Geometry: final body of the model. Coordinates: model frame, mm. Face numbers are marked on the shaded views. A direction names the side the tool comes from. Give positions to 0.01 mm unless a question says otherwise; leave off trailing zeros. Write each loop counter-clockwise with the first axis right and the second up, starting at its lowest first coordinate (ties: lowest second). Pieces come first, ordered by that corner, then holes. Notation, with made-up numbers: (1.25, -17) -> (36.25, -17) arc R15 ccw to (36.25, 11) -> close; hole circle Ø5 at (-2, 76). An arc over 180 degrees is marked (long way). Use CSV: the item, a comma, the result in double quotes. Start each with the question number.
1) Section C-C (x = -1.75). Output: boundary loops of the cut face in (y, z).
2) Section A-A (x = -12.5). Output: boundary loops of the cut face in (y, z).
3) Section D-D (z = -1). Output: boundary loops of the cut face in (x, y).
4) Set-up query: the marked faces 1 and 2. Return all of +Z, -Z, +X, -X, +Y, -Y with unobstructed straight access to the full face (end or side cutting, diameter ignored); none if empty.
5) Section B-B (y = 17.5). Output: boundary loops of the cut face in (x, z), plus the area to 3 significant figures.
6) Material intervals for line 1 (Y direction, x = -12.5, z = -2.3); line 2 (Y direction, x = -12.5, z = -1.5); line 3 (Z direction, x = -18.25, y = 10), sorted ascending. Write a range as [from, to].
7) Contact query for flat-ended pins moving along their axis: P1, Ø2, axis at x = -18, z = -9, coming from the +Y side; P2, Ø3, axis at x = -5.5, y = 11.5, coming from the -Z side; P3, Ø5, axis at x = -17.5, z = -2, coming from the +Y side; P4, Ø1, axis at x = -11, z = -6, coming from the +Y side. Output: stop coordinate, or through.
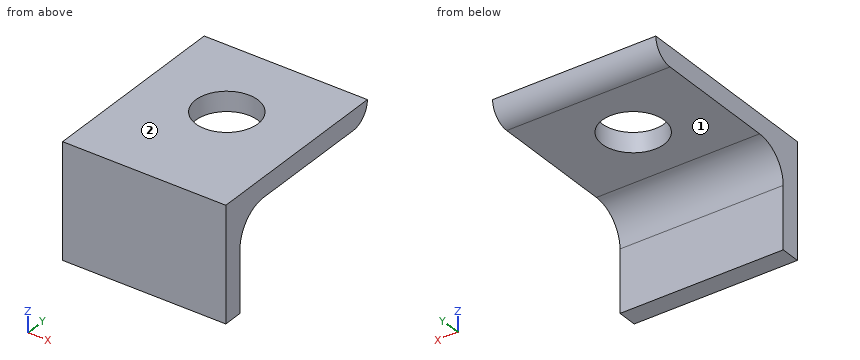
```python
from build123d import *

# Parameters (mm, degrees)
L_ANGLE_EQUAL_30X30X3_2_DEPTH  = 25
F_9_5_9_5_DIAMETER_HOLE1_D     = 9.5
F_9_5_9_5_DIAMETER_HOLE1_DEPTH = 18
F_9_5_9_5_DIAMETER_HOLE1_TIP   = 2.85408794
CUT_EXTRUDE1_REACH             = 51.244
SKETCH15_W                     = 25
SKETCH15_H                     = 12.5


with BuildPart() as part:
    # Sketch19 → L angle (equal) 30X30X3(2) (new body)
    with BuildSketch(Plane(origin=(-25, 0, 0), x_dir=(0, 0, -1), z_dir=(1, 0, 0))):
        with BuildLine():
            Line((0, 30), (0, 0))
            Line((0, 0), (30, 0))
            ThreePointArc((30, 0), (29.121320344, 2.121320344), (27, 3))
            Line((27, 3), (8, 3))
            ThreePointArc((8, 3), (4.464466094, 4.464466094), (3, 8))
            Line((3, 8), (3, 27))
            ThreePointArc((3, 27), (2.121320344, 29.121320344), (0, 30))
        make_face()
    extrude(amount=L_ANGLE_EQUAL_30X30X3_2_DEPTH)

    # Ø9.5 (9.5) Diameter Hole1
    with Locations(Plane(origin=(0, 0, -3), x_dir=(-1, 0, 0), z_dir=(0, 0, -1))):
        with Locations((12.5, 17.5)):
            Hole(F_9_5_9_5_DIAMETER_HOLE1_D / 2, depth=F_9_5_9_5_DIAMETER_HOLE1_DEPTH)
            with Locations((0, 0, -(F_9_5_9_5_DIAMETER_HOLE1_DEPTH + F_9_5_9_5_DIAMETER_HOLE1_TIP / 2))):  # 118° drill point
                Cone(0, F_9_5_9_5_DIAMETER_HOLE1_D / 2, F_9_5_9_5_DIAMETER_HOLE1_TIP, mode=Mode.SUBTRACT)

    # Sketch15 → Cut-Extrude1 (cut, up to next)
    with BuildSketch(Plane.XZ, mode=Mode.PRIVATE) as cut_extrude1_sk1:
        with Locations((-12.5, -23.75)):
            Rectangle(SKETCH15_W, SKETCH15_H)
    cut_extrude1_tool1 = extrude(cut_extrude1_sk1.sketch, amount=-CUT_EXTRUDE1_REACH, mode=Mode.PRIVATE) & part.part
    add(cut_extrude1_tool1.solids().sort_by_distance((-12.5, 0, -23.75))[0], mode=Mode.SUBTRACT)


solid = part.part
```
Answers follow:
1,outline,"(0, -17.5) -> (3, -17.5) -> (3, -8) arc R5 cw to (8, -3) -> (27, -3) arc R3 ccw to (30, 0) -> (0, 0) -> close"
2,outline,"(0, -17.5) -> (3, -17.5) -> (3, -8) arc R5 cw to (8, -3) -> (12.75, -3) -> (12.75, 0) -> (0, 0) -> close; (22.25, -3) -> (27, -3) arc R3 ccw to (30, 0) -> (22.25, 0) -> close"
3,outline,"(-25, 0) -> (0, 0) -> (0, 29.83) -> (-25, 29.83) -> close; hole circle Ø9.5 at (-12.5, 17.5)"
4,face 1,"-Z, +X, -X, +Y"
4,face 2,"+Z, +X, -X, +Y, -Y"
5,outline,"(-25, -3) -> (-17.25, -3) -> (-17.25, 0) -> (-25, 0) -> close; (-7.75, -3) -> (0, -3) -> (0, 0) -> (-7.75, 0) -> close"
5,area,"46.5 mm^2"
6,line 1,"y = [0, 12.75], [22.25, 28.93]"
6,line 2,"y = [0, 12.75], [22.25, 29.6]"
6,line 3,"z = [-3, 0]"
7,P1,"stops at y = 3"
7,P2,"stops at z = -3"
7,P3,"stops at y = 30"
7,P4,"stops at y = 3.67"
